Source: CAD feature listing. Evaluate the final solid. Frame: model axes, mm. A direction names the side the tool comes from. Round coordinates to 2 decimals unless told otherwise and drop trailing zeros. Order: outer loops, then holes, each group sorted by start corner. A loop starts at its lowest first (then second) coordinate and runs counter-clockwise, first axis right, second up. Notation, with made-up numbers: (-38.75, 23.25) -> (6.25, 23.25) arc R16 ccw to (6.25, 48.25) -> close; hole circle Ø4 at (-14.5, 51.5). An arc over 180 degrees is marked (long way). Answer as CSV lines item,"result".
from build123d import *

# Parameters (mm, degrees)
SKETCH1_W           = 6.9
SKETCH1_H           = 9
BOSS_EXTRUDE1_DEPTH = 2.3
SKETCH2_W           = 0.964703619
SKETCH2_H           = 2.203085013
BOSS_EXTRUDE2_DEPTH = 1.3
SKETCH3_W           = 0.964703619
SKETCH3_H           = 2.203085013
BOSS_EXTRUDE3_DEPTH = 0.0001


with BuildPart() as part:
    # Sketch1 → Boss-Extrude1 (new body)
    with BuildSketch(Plane.XY):
        Rectangle(SKETCH1_W, SKETCH1_H)
    extrude(amount=BOSS_EXTRUDE1_DEPTH)

    # Sketch2 → Boss-Extrude2 (add)
    with BuildSketch(Plane(origin=(0, 0, 0), x_dir=(-1, 0, 0), z_dir=(0, 0, -1))):
        Polygon((3.25, 4.5), (3.25, 5.020423263), (2.54, 5.730423263), (-2.54, 5.730423263), (-3.25, 5.020423263), (-3.25, 4.5), align=None)
        with Locations((-2.667648191, -5.601542507)):
            Rectangle(SKETCH2_W, SKETCH2_H)
        with Locations((2.667648191, -5.601542507)):
            Rectangle(SKETCH2_W, SKETCH2_H)
    extrude(amount=-BOSS_EXTRUDE2_DEPTH)

    # Sketch3 → Boss-Extrude3 (add)
    with BuildSketch(Plane(origin=(0, 0, 0), x_dir=(-1, 0, 0), z_dir=(0, 0, -1))):
        Polygon((-3.25, 4.5), (-3.25, 5.020423263), (-2.54, 5.730423263), (2.54, 5.730423263), (3.25, 5.020423263), (3.25, 4.5), align=None)
        with Locations((-2.667648191, -5.601542507)):
            Rectangle(SKETCH3_W, SKETCH3_H)
        with Locations((2.667648191, -5.601542507)):
            Rectangle(SKETCH3_W, SKETCH3_H)
    extrude(amount=BOSS_EXTRUDE3_DEPTH)


solid = part.part
1. Reachability of faces 4 (the flat face through (0, 5, 1.3)), 5 (the flat face through (2.185, -6, 1)), 6 (the flat face through (3, -6, 1.3)), 7 (the flat face through (0, 5, 0)), 8 (the flat face through (-3.15, -6, 1)) from +Z, -Z, +X, -X, +Y, -Y: full face, straight path, thin tool, end or side. Return the list, or none.
Results below:
face 4,"+Z, +X, -X, +Y"
face 5,"+Z, -Z, -Y"
face 6,"+Z, +X, -X, -Y"
face 7,"-Z, +X, -X, +Y, -Y"
face 8,"+Z, -Z, -X, -Y"
2. Section query A-A on z = 1. Return loops of the section in (x, y).
Results below:
outline,"(-3.45, -4.5) -> (-3.15, -4.5) -> (-3.15, -6.7) -> (-2.19, -6.7) -> (-2.19, -4.5) -> (2.19, -4.5) -> (2.19, -6.7) -> (3.15, -6.7) -> (3.15, -4.5) -> (3.45, -4.5) -> (3.45, 4.5) -> (3.25, 4.5) -> (3.25, 5.02) -> (2.54, 5.73) -> (-2.54, 5.73) -> (-3.25, 5.02) -> (-3.25, 4.5) -> (-3.45, 4.5) -> close"
3. Pin query (flat end, axial travel): pin 1 (0.7 mm diameter, centred on y = -6, z = 1, fed in from +X); pin 2 (0.7 mm diameter, centred on y = -6, z = 0.5, fed in from -X); pin 3 (0.6 mm diameter, centred on x = -0.5, y = 5, fed in from +Z). Return the tip coordinate at first contact, or that it passes through.
Results below:
pin 1,"x = 3.15"
pin 2,"x = -3.15"
pin 3,"z = 1.3"
4. Mould query, pull axis X, two halves, no side actions, for faces 1 (the flat face through (-3.45, 0, 1)), 2 (the flat face through (-3, -6, 0)), 3 (the flat face through (0, -4.5, 1)). Classes: released by +X, released by -X, zero draft, split by the parting line, or undercut.
Results below:
face 1,"released by -X"
face 2,"zero draft"
face 3,"undercut"
5. Line query: L1, parallel to Y at x = 1.75, z = 0.55; L2, parallel to Z at x = 0.75, y = 4.75; L3, parallel to Y at x = 3, z = 1.65. Output: solid intervals per line, ascending. Write a range as [from, to].
Results below:
L1,"[-4.5, 5.73]"
L2,"[0, 1.3]"
L3,"[-4.5, 4.5]"
